Check sheet for the modelled part. Datum: model origin and axes. Units: mm. A direction names the side the tool comes from. Give positions to 0.01 mm unless a question says otherwise; leave off trailing zeros. Order: outer loops, then holes, each group sorted by start corner. A loop starts at its lowest first (then second) coordinate and runs counter-clockwise, first axis right, second up. Notation, with made-up numbers: (84.25, -12) -> (97.25, -12) arc R30 ccw to (97.25, 21) -> close; hole circle Ø8 at (7.25, 65.25). An arc over 180 degrees is marked (long way). Write each question's results on one line, items separated by ' | '.
from build123d import *

# Parameters (mm, degrees)
F0_W     = 30
F0_H     = 30
F1_DEPTH = 35
F2_DEPTH = 30
F3_R     = 2.5
F4_DEPTH = 35.001
F5_W     = 30
F5_H     = 30
F5_R     = 12.5
F6_DEPTH = 30


with BuildPart() as f1:
    # F0 (on Top) → F1 (new body)
    with BuildSketch(Plane.XY):
        Rectangle(F0_W, F0_H)
        with BuildLine():
            ThreePointArc((-2.5, -6.5383484153), (-3.9686269666, 5.7662812973), (7, 0))
            ThreePointArc((7, 0), (5.7662812973, -3.9686269666), (2.5, -6.5383484153))
            Line((2.5, -6.5383484153), (2.5, -9.5))
            Line((2.5, -9.5), (0, -9.5))
            Line((0, -9.5), (-2.5, -9.5))
            Line((-2.5, -9.5), (-2.5, -6.5383484153))
        make_face(mode=Mode.SUBTRACT)
        with BuildLine():
            ThreePointArc((2.5, -6.5383484153), (5.7662812973, -3.9686269666), (7, 0))
            ThreePointArc((7, 0), (-3.9686269666, 5.7662812973), (-2.5, -6.5383484153))
            ThreePointArc((-2.5, -6.5383484153), (0, -7), (2.5, -6.5383484153))
        make_face()
        with BuildLine():
            ThreePointArc((2.5, -6.5383484153), (0, -7), (-2.5, -6.5383484153))
            Line((-2.5, -6.5383484153), (-2.5, -9.5))
            Line((-2.5, -9.5), (0, -9.5))
            Line((0, -9.5), (2.5, -9.5))
            Line((2.5, -9.5), (2.5, -6.5383484153))
        make_face()
    extrude(amount=F1_DEPTH)

    # F0 (on Top) → F2 (cut)
    with BuildSketch(Plane.XY):
        with BuildLine():
            ThreePointArc((2.5, -6.5383484153), (5.7662812973, -3.9686269666), (7, 0))
            ThreePointArc((7, 0), (-3.9686269666, 5.7662812973), (-2.5, -6.5383484153))
            ThreePointArc((-2.5, -6.5383484153), (0, -7), (2.5, -6.5383484153))
        make_face()
        with BuildLine():
            ThreePointArc((2.5, -6.5383484153), (0, -7), (-2.5, -6.5383484153))
            Line((-2.5, -6.5383484153), (-2.5, -9.5))
            Line((-2.5, -9.5), (0, -9.5))
            Line((0, -9.5), (2.5, -9.5))
            Line((2.5, -9.5), (2.5, -6.5383484153))
        make_face()
    extrude(amount=F2_DEPTH, mode=Mode.SUBTRACT)

    # F3 (on face) → F4 (cut, through all)
    with BuildSketch(Plane.XY.offset(35)):
        Circle(F3_R)
    extrude(amount=-F4_DEPTH, mode=Mode.SUBTRACT)

    # F5 (on face) → F6 (cut)
    with BuildSketch(Plane.XY):
        Rectangle(F5_W, F5_H)
        Circle(F5_R, mode=Mode.SUBTRACT)
    extrude(amount=F6_DEPTH, mode=Mode.SUBTRACT)


solid = f1.part
1. Mould release check, pull along X, two halves, no side actions. Record for faces 1 (the flat face through (0, -9.5, 15)), 2 (the flat face through (-2.5, -8, 15)), 3 (the flat face through (-15, 0, 32)), 4 (the flat face through (0, -15, 32)): +X half, -X half, draft (parallel to the pull), parting line (faces both ways), or undercut.
Verdict:
face 1: undercut | face 2: undercut | face 3: -X half | face 4: draft
2. Material ranges on probe 1 along Y at (x, z) = (0, 33.75); probe 2 along Z at (x, y) = (-9, -9.5); probe 3 along Y at (x, z) = (0, 22.75), recorded low to high. Write a range as from..to.
Verdict:
probe 1: y = -15..-2.5, 2.5..15 | probe 2: z = 30..35 | probe 3: y = -12.5..-9.5, 7..12.5
3. Gauge pin test, flat ends, axial feed: pin 1 Ø5 at (x, z) = (-3.5, 13) entering from +Y; pin 2 Ø18 at (x, y) = (0, 0) entering from -Z; pin 3 Ø0.9 at (y, z) = (-8.5, 14.5) entering from -X; pin 4 Ø6 at (y, z) = (5, 24.5) entering from +X. Record the tip position at first contact, or that the pin passes through.
Verdict:
pin 1: stops at y = 12.46 | pin 2: stops at z = 0 | pin 3: stops at x = -9.56 | pin 4: stops at x = 12.34
4. Section check A-A on x = 0. Record the cut outline in (y, z).
Verdict:
outline: (-15, 30) -> (-12.5, 30) -> (-12.5, 0) -> (-9.5, 0) -> (-9.5, 30) -> (-2.5, 30) -> (-2.5, 35) -> (-15, 35) -> close; (2.5, 30) -> (7, 30) -> (7, 0) -> (12.5, 0) -> (12.5, 30) -> (15, 30) -> (15, 35) -> (2.5, 35) -> close
5. Access from +Z, -Z, +X, -X, +Y, -Y to the whole of each face (thin tool, end or side, straight path). Record for faces 5 (the flat face through (-4, 0, 35)), 6 (the cylindrical face through (11.923, 3.755, 14.79)).
Verdict:
face 5: +Z, +X, -X, +Y, -Y | face 6: -Z
6. Section check C-C on z = 15.5. Record the cut outline in (x, y), then the cut area to 3 significant figures.
Verdict:
outline: circle Ø25 at (0, 0); hole (-2.5, -9.5) -> (2.5, -9.5) -> (2.5, -6.54) arc R7 ccw (long way) to (-2.5, -6.54) -> close | area: 324 mm^2
7. Section check B-B on y = 1.25. Record the cut outline in (x, z).
Verdict:
outline: (-15, 30) -> (-12.44, 30) -> (-12.44, 0) -> (-6.89, 0) -> (-6.89, 30) -> (-2.17, 30) -> (-2.17, 35) -> (-15, 35) -> close; (2.17, 30) -> (6.89, 30) -> (6.89, 0) -> (12.44, 0) -> (12.44, 30) -> (15, 30) -> (15, 35) -> (2.17, 35) -> close
8. Section check D-D on x = -3.25. Record the cut outline in (y, z), then the cut area to 3 significant figures.
Verdict:
outline: (-15, 30) -> (-12.07, 30) -> (-12.07, 0) -> (-6.2, 0) -> (-6.2, 30) -> (6.2, 30) -> (6.2, 0) -> (12.07, 0) -> (12.07, 30) -> (15, 30) -> (15, 35) -> (-15, 35) -> close | area: 502 mm^2
